Geometry: final body of the model. Coordinates: model frame, mm. A direction names the side the tool comes from. Round coordinates to 2 decimals unless told otherwise and drop trailing zeros. Loops run counter-clockwise (first coordinate to the right, second up) from the corner with the lowest first, then second, coordinate; pieces in that order, holes last. Notation, with made-up numbers: M 61.5,-12.5 L 68.5,-12.5 A26 cw 68.5,5.5 Z; hole C 74.5,52.5 d2. An arc over 180 degrees is marked long. Answer as a JSON object with one key per item and string values.
Autodesk Inventor part; units mm, degrees
ref_plane "YZ Plane" through (0, 0, 0) normal (1, 0, 0) x (0, 1, 0)
ref_plane "XZ Plane" through (0, 0, 0) normal (0, 1, 0) x (-1, 0, 0)
ref_plane "XY Plane" through (0, 0, 0) normal (0, 0, 1) x (1, 0, 0)
sketch "Sketch1" plane through (0, 0, 0) normal (0, 1, 0) x (-1, 0, 0)
  line L0 (0, 0) -> (60, 0) construction
  line L1 (60, 0) -> (60, -25) construction
  line L2 (60, -25) -> (0, -25) construction
  line L3 (0, -25) -> (0, 0) construction
  line L4 (60.5, 0.5) -> (-0.5, 0.5)
  line L5 (-0.5, 0.5) -> (-0.5, -25.5)
  line L6 (-0.5, -25.5) -> (60.5, -25.5)
  line L7 (60.5, -25.5) -> (60.5, 0.5)
  circle A0 centre (53, -19) radius 1.8
  circle A1 centre (7, -19) radius 1.8
  circle A2 centre (7, -6) radius 1.8
  circle A3 centre (53, -6) radius 1.8
  line L8 (53, -19) -> (7, -19) construction
  line L9 (7, -19) -> (7, -6) construction
  point P0 (30, -19)
  point P1 (30, -25)
  point P2 (7, -12.5)
  point P3 (0, -12.5)
  dimension "d0" = 25
  dimension "d1" = 60
  dimension "d2" = 0.5
  dimension "d3" = 0.5
  dimension "d4" = 0.5
  dimension "d5" = 0.5
  dimension "d6" = 3.6
  dimension "d7" = 46
  dimension "d8" = 13
sketch "Sketch2" plane through (0, 0, 0) normal (0, 1, 0) x (-1, 0, 0)
  line L0 (-5.4, 5) -> (65.4, 5)
  line L1 (65.4, 5) -> (65.4, -30)
  line L2 (65.4, -30) -> (-5.4, -30)
  line L3 (-5.4, -30) -> (-5.4, 5)
  line L4 (60.5, -25.5) -> (60.5, 0.5) construction
  line L5 (-0.5, 0.5) -> (-0.5, -25.5) construction
  line L6 (-0.5, -25.5) -> (60.5, -25.5) construction
  point P0 (0, 0)
  point P1 (60.5, -12.5)
  point P2 (65.4, -12.5)
  point P3 (30, -25.5)
  point P4 (30, -30)
  dimension "d9" = 70.8
  dimension "d10" = 35
extrude "Extrusion1" add sketch "Sketch2" along normal blind 10 and the other way blind 35.4
extrude "Extrusion2" cut sketch "Sketch1" along normal blind 10 and the other way blind 2
extrude "Extrusion3" cut sketch "Sketch1" along normal blind 10 and the other way blind 30.4 contours A0 | A1 | A2 | A3
sketch "Sketch3" plane through (5.4, 10, -30) normal (0, 0, -1) x (-1, 0, 0)
  line L0 (70.8, -45.4) -> (0, -45.4)
  line L1 (0, -45.4) -> (0, -75.4)
  line L2 (0, -75.4) -> (10, -75.4)
  line L3 (10, -75.4) -> (10, -48.575)
  line L4 (13.175, -45.4) -> (57.625, -45.4)
  line L5 (60.8, -48.575) -> (60.8, -75.4)
  line L6 (60.8, -75.4) -> (70.8, -75.4)
  line L7 (70.8, -75.4) -> (70.8, -45.4)
  arc A0 (13.175, -45.4) -> (10, -48.575) centre (13.175, -48.575) ccw
  arc A1 (60.8, -48.575) -> (57.625, -45.4) centre (57.625, -48.575) ccw
  point P0 (5.4, -10)
  point P1 (10, -45.4)
  point P2 (60.8, -45.4)
  point P3 (35.4, -45.4)
  point P4 (13.175, -45.4)
  point P5 (57.625, -45.4)
  dimension "d23" = 50.8
  dimension "d24" = 3.175
  dimension "d25" = 10
  dimension "d26" = 30
extrude "Extrusion4" add sketch "Sketch3" against normal up to surface (35 mm away)
sketch "Sketch4" plane through (0, -2, 0) normal (0, 1, 0) x (1, 0, 0)
  circle A0 centre (-42.5, 12.5) radius 3
  circle A1 centre (-17.5, 12.5) radius 3
  line L0 (-60.5, 25.5) -> (0.5, 25.5) construction
  line L1 (-60.5, -0.5) -> (-60.5, 25.5) construction
  line L2 (-42.5, 12.5) -> (-17.5, 12.5) construction
  point P0 (0, 0)
  point P1 (-30, 25.5)
  point P2 (-30, 12.5)
  point P3 (-60.5, 12.5)
  dimension "d29" = 6
  dimension "d30" = 25
extrude "Extrusion5" cut sketch "Sketch4" against normal up to surface (33.4 mm away)
sketch "Sketch5" plane through (0, -2, 0) normal (0, 1, 0) x (1, 0, 0)
  circle A0 centre (-42.5, 12.5) radius 3 construction
  circle A1 centre (-17.5, 12.5) radius 3 construction
  circle A2 centre (-17.5, 12.5) radius 6
  circle A3 centre (-42.5, 12.5) radius 6
  point P0 (0, 0)
  dimension "d34" = 12
extrude "Extrusion6" cut sketch "Sketch5" against normal blind 10
fillet "Fillet1" radius 2 2 edges at (-65.4, 10, -12.5) (5.4, 10, -12.5)
fillet "Fillet2" radius 2 2 edges at (-65.4, -65.4, -12.5) (5.4, -65.4, -12.5)
sketch "Sketch6" plane through (-52.225, -35.4, 5) normal (0, 0, 1) x (1, 0, 0)
  line L0 (44.45, 0) -> (0, 0) construction
  line L1 (4.725, 38.4) -> (39.725, 38.4)
  line L2 (44.45, 0) -> (0, 0)
  line L3 (-11.175, 45.4) -> (55.625, 45.4)
  line L4 (39.725, 38.4) -> (39.725, 45.4)
  line L5 (4.725, 38.4) -> (4.725, 45.4)
  point P0 (52.225, 35.4)
  point P1 (22.225, 38.4)
  point P2 (22.225, 0)
  point P3 (70.325, 0)
  point P4 (-0.475, 0)
  dimension "d39" = 38.4
  dimension "d40" = 35
extrude "Extrusion7" cut sketch "Sketch6" against normal up to surface (4.5 mm away)
sketch "Sketch7" plane through (-4.6, -65.4, -30) normal (0, 0, -1) x (-1, 0, 0)
  arc A0 (5.8041, 75.4) -> (44.9959, 75.4) centre (25.4, 85.4) ccw
  line L0 (-8, 75.4) -> (58.8, 75.4)
  point P0 (-4.6, 65.4)
  point P1 (25.4, 75.4)
  dimension "d44" = 22
  dimension "d45" = 10
extrude "Extrusion8" cut sketch "Sketch7" against normal blind 10
properties part number "BK12_Spacer"
1) Section query B-B (z = -12.5). Count the separate pieces of the cut face and the enclosed holes in it, and give its area (3 significant figures).
Results:
{"separate pieces": "3", "enclosed holes": "0", "area": "2,560 mm2"}
2) Ray query, line 1 (Z direction, x = -7, y = -22.75); line 2 (X direction, y = -20, z = -12.5); line 3 (Z direction, x = -42.5, y = -27.5). Return the intervals inside material, ascending.
Results:
{"line 1": "-30 to -20.8, -17.2 to -7.8, -4.2 to 5", "line 2": "-65.4 to -45.5, -39.5 to -20.5, -14.5 to 5.4", "line 3": "-30 to -15.5, -9.5 to 5"}
3) Reachability of faces 1 (the cylindrical face through (-52.766, -16.001, -17.215)), 2 (the cylindrical face through (-5.55, -36.31, -12.74)), 3 (the flat face through (-30, 3, 3)) from +Z, -Z, +X, -X, +Y, -Y: full face, straight path, thin tool, end or side. Return the list, or none.
Results:
{"face 1": "+Y", "face 2": "+Z, -Z, -Y", "face 3": "+Z, +Y"}
4) Section query A-A (y = -42.5). Return the cut outline in (x, z), and give its area (3 significant figures).
Results:
{"outline": "M -65.4,-30 L -55.4,-30 L -55.4,5 L -65.4,5 Z; M -4.6,-30 L 5.4,-30 L 5.4,5 L -4.6,5 Z", "area": "700 mm2"}
5) Pin query (flat end, axial travel): P1, Ø1, axis at x = -29, z = -25.5, coming from the -Y side; P2, Ø6, axis at x = -19, z = -13.5, coming from the +Y side; P3, Ø4.5, axis at x = -53, z = -19, coming from the +Y side; P4, Ø6, axis at x = -43, y = 7, coming from the -Z side. Return the tip coordinate at first contact, or that it passes through.
Results:
{"P1": "y = -35.4", "P2": "y = -12", "P3": "y = -2", "P4": "through"}
6) Section query C-C (z = -1). Return the cut outline in (x, y) (3 decimals), and give its area (3 significant figures).
Results:
{"outline": "M -65.4,-63.4 A2 ccw -63.4,-65.4 L -55.4,-65.4 L -55.4,-38.575 A3.175 cw -52.225,-35.4 L -7.775,-35.4 A3.175 cw -4.6,-38.575 L -4.6,-65.4 L 3.4,-65.4 A2 ccw 5.4,-63.4 L 5.4,8 A2 ccw 3.4,10 L 0.5,10 L 0.5,-2 L -60.5,-2 L -60.5,10 L -63.4,10 A2 ccw -65.4,8 Z", "area": "3,080 mm2"}
7) Section query D-D (x = -17.5). Return the cut outline in (y, z), and give its area (3 significant figures).
Results:
{"outline": "M -35.4,-30 L 1.9,-30 L 1.9,-25.5 L -2,-25.5 L -2,-18.5 L -12,-18.5 L -12,-15.5 L -35.4,-15.5 Z; M -35.4,-9.5 L -12,-9.5 L -12,-6.5 L -2,-6.5 L -2,0.5 L 3,0.5 L 3,5 L -35.4,5 Z", "area": "949 mm2"}
8) Pull-direction query (X, two-part tool) for faces 4 (the flat face through (-4.6, -52, -13)), 5 (the flat face through (-1, -65.4, -13)), 6 (the flat face through (-65.4, -28, -12)); classes: +X half, -X half, draft (parallel to the pull), parting line (faces both ways), or undercut.
Results:
{"face 4": "undercut", "face 5": "draft", "face 6": "-X half"}
